Input: dimensioned drawing with shaded views. Units: mm. Origin: part minimum x, y, z. A direction names the side the tool comes from. Round coordinates to 2 decimals unless told otherwise and drop trailing zeros. Loops run counter-clockwise (first coordinate to the right, second up) from the corner with the lowest first, then second, coordinate; pieces in that order, holes last. Notation, with made-up numbers: (38.25, -21) - (74.25, -21) arc R12 cw to (74.25, 2) - close; hole circle Ø8 at (56, -1). An arc over 180 degrees is marked (long way). Answer as a JSON object with one key per item and string values. Group by question number.
Item 1: Draft query along X for the marked faces 1, 2, 3 and 4. Return one class per face: released by +X, released by -X, zero draft, split by the parting line, or undercut.
Item 2: Section B-B (y = 17.5). Return the cut outline in (x, z).
Item 3: Line query: line 1 (X direction, y = 17.5, z = 3); line 2 (X direction, y = 10.5, z = 1); line 3 (Y direction, x = 50, z = 3.25). Output: solid intervals per line, ascending.
Item 4: Section C-C (x = 10). Return the cut outline in (y, z).
Item 5: Section A-A (z = 3.25). Return the cut outline in (x, y) (3 decimals).
Item 6: Reachability of the marked faces 5 and 6 from +Z, -Z, +X, -X, +Y, -Y: full face, straight path, thin tool, end or side. Return the list, or none.
Item 7: Section D-D (x = 54). Return the cut outline in (y, z).
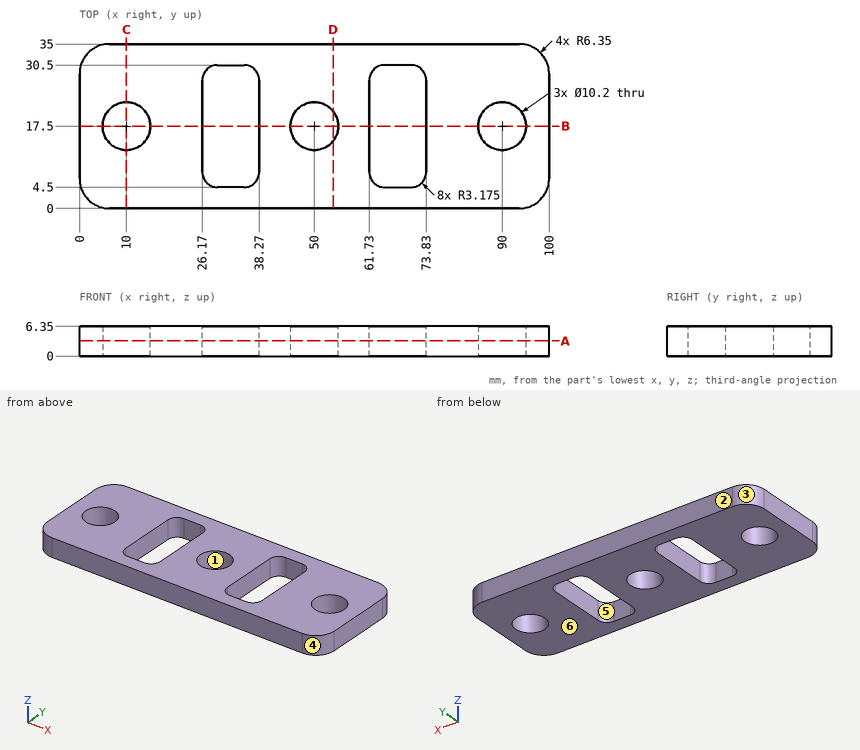
Values:
{
 "1": {"face 1": "undercut", "face 2": "zero draft", "face 3": "released by -X", "face 4": "released by +X"},
 "2": {"outline": "(0, 0) - (4.9, 0) - (4.9, 6.35) - (0, 6.35) - close; (15.1, 0) - (26.17, 0) - (26.17, 6.35) - (15.1, 6.35) - close; (38.27, 0) - (44.9, 0) - (44.9, 6.35) - (38.27, 6.35) - close; (55.1, 0) - (61.73, 0) - (61.73, 6.35) - (55.1, 6.35) - close; (73.83, 0) - (84.9, 0) - (84.9, 6.35) - (73.83, 6.35) - close; (95.1, 0) - (100, 0) - (100, 6.35) - (95.1, 6.35) - close"},
 "3": {"line 1": "x = 0 to 4.9, 15.1 to 26.17, 38.27 to 44.9, 55.1 to 61.73, 73.83 to 84.9, 95.1 to 100", "line 2": "x = 0 to 26.17, 38.27 to 61.73, 73.83 to 100", "line 3": "y = 0 to 12.4, 22.6 to 35"},
 "4": {"outline": "(0, 0) - (12.4, 0) - (12.4, 6.35) - (0, 6.35) - close; (22.6, 0) - (35, 0) - (35, 6.35) - (22.6, 6.35) - close"},
 "5": {"outline": "(0, 6.35) arc R6.35 ccw to (6.35, 0) - (93.65, 0) arc R6.35 ccw to (100, 6.35) - (100, 28.65) arc R6.35 ccw to (93.65, 35) - (6.35, 35) arc R6.35 ccw to (0, 28.65) - close; hole circle Ø10.2 at (10, 17.5); hole (26.17, 7.675) arc R3.175 ccw to (29.345, 4.5) - (35.095, 4.5) arc R3.175 ccw to (38.27, 7.675) - (38.27, 27.325) arc R3.175 ccw to (35.095, 30.5) - (29.345, 30.5) arc R3.175 ccw to (26.17, 27.325) - close; hole circle Ø10.2 at (50, 17.5); hole (61.73, 7.675) arc R3.175 ccw to (64.905, 4.5) - (70.655, 4.5) arc R3.175 ccw to (73.83, 7.675) - (73.83, 27.325) arc R3.175 ccw to (70.655, 30.5) - (64.905, 30.5) arc R3.175 ccw to (61.73, 27.325) - close; hole circle Ø10.2 at (90, 17.5)"},
 "6": {"face 5": "+Z, -Z", "face 6": "-Z, +X, -X, +Y, -Y"},
 "7": {"outline": "(0, 0) - (14.34, 0) - (14.34, 6.35) - (0, 6.35) - close; (20.66, 0) - (35, 0) - (35, 6.35) - (20.66, 6.35) - close"}
}
